The model under review builds one solid part; all positions refer to its coordinate system, in mm. Coordinates: 2 decimals unless noted, no trailing zeros. Order: outer loops, then holes, each group sorted by start corner. A loop starts at its lowest first (then second) coordinate and runs counter-clockwise, first axis right, second up. Notation, with made-up numbers: M 50.25,68 L 92.25,68 A29 ccw 92.25,91 Z; hole C -32.75,70.25 d2. An arc over 180 degrees is marked long. Answer in a Markdown table with one row per item.
from build123d import *

# Parameters (mm, degrees)
SKETCH1_R           = 10
BOSS_EXTRUDE1_DEPTH = 10
SKETCH1_2_R         = 10
BOSS_EXTRUDE2_DEPTH = 20


with BuildPart() as part:
    # Sketch1 → Boss-Extrude1 (new body)
    with BuildSketch(Plane.XY):
        with BuildLine():
            Line((-60, 20), (60, 20))
            ThreePointArc((60, 20), (80, 0), (60, -20))
            Line((60, -20), (-60, -20))
            ThreePointArc((-60, -20), (-80, 0), (-60, 20))
        make_face()
        with Locations((-60, 0)):
            Circle(SKETCH1_R, mode=Mode.SUBTRACT)
        with Locations((60, 0)):
            Circle(SKETCH1_R, mode=Mode.SUBTRACT)
    extrude(amount=BOSS_EXTRUDE1_DEPTH)

    # Sketch1<2> → Boss-Extrude2 (add)
    with BuildSketch(Plane.XY):
        with Locations((60, 0)):
            Circle(SKETCH1_2_R)
    extrude(amount=BOSS_EXTRUDE2_DEPTH)


solid = part.part
(1) Insertion check: P1, Ø16, axis at x = -60, y = 0, coming from the -Z side; P2, Ø6, axis at x = 9, y = -12, coming from the +Z side; P3, Ø6, axis at y = 15.5, z = 12.5, coming from the +X side. Each pin has a flat end and moves straight along its axis. Give the tip position at first contact, or say it passes through.
Report:
| item | result |
|---|---|
| P1 | through |
| P2 | z = 10 |
| P3 | x = 74.44 |
(2) Take a section at D-D (z = 16). Write out the cut boundary in (x, y).
Report:
| item | result |
|---|---|
| outline | C 60,0 d20 |
(3) To check wall thickness, follow line 1 (Y direction, x = -60, z = 2.5); line 2 (Z direction, x = 49.5, y = -3.5); line 3 (X direction, y = 1, z = 1). State the ranges of each line that lie inside material, in increasing order. Write a range as [from, to].
Report:
| item | result |
|---|---|
| line 1 | [-20, -10], [10, 20] |
| line 2 | [0, 10] |
| line 3 | [-79.97, -69.95], [-50.05, 79.97] |
(4) Take a section at A-A (y = 0). Write out the cut boundary in (x, z), then the cut area to 3 significant figures.
Report:
| item | result |
|---|---|
| outline | M -80,0 L -70,0 L -70,10 L -80,10 Z; M -50,0 L 80,0 L 80,10 L 70,10 L 70,20 L 50,20 L 50,10 L -50,10 Z |
| area | 1,600 mm^2 |
(5) The part is to be moulded in two halves that separate along X. For faces 1 (the cylindrical face through (-80, 0, 5)), 2 (the cylindrical face through (50, 0, 15)), 3 (the cylindrical face through (-70, 0, 5)), 4 (the flat face through (1, -20, 5)), say which applies: +X half, -X half, draft (parallel to the pull), parting line (faces both ways), or undercut.
Report:
| item | result |
|---|---|
| face 1 | -X half |
| face 2 | parting line |
| face 3 | undercut |
| face 4 | draft |
(6) Take a section at B-B (z = 7). Write out the cut boundary in (x, y), then the cut area to 3 significant figures.
Report:
| item | result |
|---|---|
| outline | M -60,-20 L 60,-20 A20 ccw 60,20 L -60,20 A20 ccw Z; hole C -60,0 d20 |
| area | 5,740 mm^2 |
(7) Take a section at C-C (x = -51.5). Write out the cut boundary in (y, z), then the cut area to 3 significant figures.
Report:
| item | result |
|---|---|
| outline | M -20,0 L -5.27,0 L -5.27,10 L -20,10 Z; M 5.27,0 L 20,0 L 20,10 L 5.27,10 Z |
| area | 295 mm^2 |
